Geometry check sheet. Reference: the model listing, model coordinates, mm. A direction names the side the tool comes from. Coordinates: 2 decimals unless noted, no trailing zeros. Order: outer loops, then holes, each group sorted by start corner. A loop starts at its lowest first (then second) coordinate and runs counter-clockwise, first axis right, second up. Notation, with made-up numbers: (6.25, 70.25) -> (40.25, 70.25) arc R22 ccw to (40.25, 108.25) -> close; hole circle Ø10 at (-28.75, 15). An arc over 180 degrees is marked (long way). Answer as CSV lines item,"result". Start each with the question number.
from build123d import *

# Parameters (mm, degrees)
BOSS_EXTRUDE1_DEPTH     = 40
CUT_EXTRUDE1_DEPTH      = 1.25
CUT_EXTRUDE1_DEPTH_BACK = 1.25


with BuildPart() as part:
    # Sketch1 → Boss-Extrude1 (new body)
    with BuildSketch(Plane.XY):
        with BuildLine():
            Line((-18.982831897, 2.385797253), (-16.305815663, 5.062813487))
            ThreePointArc((-16.305815663, 5.062813487), (-14.5, 0), (-16.305815663, -5.062813487))
            Line((-16.305815663, -5.062813487), (-18.982831897, -2.385797253))
            ThreePointArc((-18.982831897, -2.385797253), (-19.49479618, -3.00520382), (-20.114202747, -3.517168103))
            Line((-20.114202747, -3.517168103), (-16.01728135, -7.6140895))
            Line((-16.01728135, -7.6140895), (16.01728135, -7.6140895))
            Line((16.01728135, -7.6140895), (20.114202747, -3.517168103))
            ThreePointArc((20.114202747, -3.517168103), (19.49479618, -3.00520382), (18.982831897, -2.385797253))
            Line((18.982831897, -2.385797253), (16.305815663, -5.062813487))
            ThreePointArc((16.305815663, -5.062813487), (14.5, 0), (16.305815663, 5.062813487))
            Line((16.305815663, 5.062813487), (18.982831897, 2.385797253))
            ThreePointArc((18.982831897, 2.385797253), (19.49479618, 3.00520382), (20.114202747, 3.517168103))
            Line((20.114202747, 3.517168103), (17.437186513, 6.194184337))
            ThreePointArc((17.437186513, 6.194184337), (22.5, 8), (27.562813487, 6.194184337))
            Line((27.562813487, 6.194184337), (24.885797253, 3.517168103))
            ThreePointArc((24.885797253, 3.517168103), (25.50520382, 3.00520382), (26.017168103, 2.385797253))
            Line((26.017168103, 2.385797253), (28.694184337, 5.062813487))
            ThreePointArc((28.694184337, 5.062813487), (30.5, 0), (28.694184337, -5.062813487))
            Line((28.694184337, -5.062813487), (26.017168103, -2.385797253))
            ThreePointArc((26.017168103, -2.385797253), (25.50520382, -3.00520382), (24.885797253, -3.517168103))
            Line((24.885797253, -3.517168103), (28.98271865, -7.6140895))
            ThreePointArc((28.98271865, -7.6140895), (31.884585633, 3.453918427), (22.5, 10))
            Line((22.5, 10), (-22.5, 10))
            ThreePointArc((-22.5, 10), (-31.884585633, 3.453918427), (-28.98271865, -7.6140895))
            Line((-28.98271865, -7.6140895), (-24.885797253, -3.517168103))
            ThreePointArc((-24.885797253, -3.517168103), (-25.50520382, -3.00520382), (-26.017168103, -2.385797253))
            Line((-26.017168103, -2.385797253), (-28.694184337, -5.062813487))
            ThreePointArc((-28.694184337, -5.062813487), (-30.5, 0), (-28.694184337, 5.062813487))
            Line((-28.694184337, 5.062813487), (-26.017168103, 2.385797253))
            ThreePointArc((-26.017168103, 2.385797253), (-25.50520382, 3.00520382), (-24.885797253, 3.517168103))
            Line((-24.885797253, 3.517168103), (-27.562813487, 6.194184337))
            ThreePointArc((-27.562813487, 6.194184337), (-22.5, 8), (-17.437186513, 6.194184337))
            Line((-17.437186513, 6.194184337), (-20.114202747, 3.517168103))
            ThreePointArc((-20.114202747, 3.517168103), (-19.49479618, 3.00520382), (-18.982831897, 2.385797253))
        make_face()
    extrude(amount=BOSS_EXTRUDE1_DEPTH)

    # Sketch2 → Cut-Extrude1 (cut, two sides)
    with BuildSketch(Plane(origin=(0, 0, 0), x_dir=(0, 0, -1), z_dir=(1, 0, 0))) as cut_extrude1_sk:
        with BuildLine():
            Line((-40, 6), (-40, 8))
            ThreePointArc((-40, 8), (-38.585786438, 8.585786438), (-38, 10))
            Line((-38, 10), (-36, 10))
            ThreePointArc((-36, 10), (-37.171572875, 7.171572875), (-40, 6))
        make_face()
        with BuildLine():
            Line((-2, 10), (-4, 10))
            ThreePointArc((-4, 10), (-2.828427125, 7.171572875), (0, 6))
            Line((0, 6), (0, 8))
            ThreePointArc((0, 8), (-1.414213562, 8.585786438), (-2, 10))
        make_face()
    extrude(amount=CUT_EXTRUDE1_DEPTH, mode=Mode.SUBTRACT)
    extrude(cut_extrude1_sk.sketch, amount=-CUT_EXTRUDE1_DEPTH_BACK, mode=Mode.SUBTRACT)


solid = part.part
Q1. Sectioned sample at D-D, the plane y = 8.75. Record the cut outline in (x, z).
Q2. Sectioned sample at B-B, the plane y = 1. Record the cut outline in (x, z), then the cut area to 3 significant figures.
Q3. Sectioned sample at A-A, the plane x = 0. Record the cut outline in (y, z), then the cut area to 3 significant figures.
Q4. Go/stop test with flat-tipped pins: pin 1 Ø2 at (y, z) = (8.5, 37.5) entering from -X; pin 2 Ø4.5 at (y, z) = (7.5, 38.5) entering from +X; pin 3 Ø3 at (y, z) = (8.5, 1.5) entering from -X. Record where each tip stops, or that it passes through.
Q5. Thickness scan on L1, parallel to X at y = 0.5, z = 22.5; L2, parallel to X at y = 1.25, z = 22.5; L3, parallel to Y at x = 19, z = 12. Record the ranges inside material, lowest first.
Q6. Access from +Z, -Z, +X, -X, +Y, -Y to the whole of each face (thin tool, end or side, straight path). Record for faces 1 (the flat face through (-17.66, 3.71, 19.72)), 2 (the flat face through (0, 10, 20)), 3 (the flat face through (18.04, -5.59, 19.72)), 4 (the cylindrical face through (-0.018, 7.203, 37.141)).
Q7. Release check for a two-part mould opening along X. For faces 5 (the cylindrical face through (31.942, 3.293, 19.72)), 6 (the flat face through (-26.21, 4.84, 19.72)), 7 (the flat face through (26.91, -5.54, 19.72)), 8 (the flat face through (0, 1, 40)) record: released by +X, released by -X, zero draft, split by the parting line, or undercut.
Geometry results:
1,outline,"(-27.34, 0) -> (27.34, 0) -> (27.34, 40) -> (-27.34, 40) -> close; hole (-1.25, 1.56) -> (1.25, 1.56) -> (1.25, 3.8) -> (-1.25, 3.8) -> close; hole (-1.25, 36.2) -> (1.25, 36.2) -> (1.25, 38.44) -> (-1.25, 38.44) -> close"
2,outline,"(-32.45, 0) -> (-30.44, 0) -> (-30.44, 40) -> (-32.45, 40) -> close; (-14.56, 0) -> (14.56, 0) -> (14.56, 40) -> (-14.56, 40) -> close; (30.44, 0) -> (32.45, 0) -> (32.45, 40) -> (30.44, 40) -> close"
2,area,"1,330 mm^2"
3,outline,"(-7.61, 0) -> (6, 0) arc R4 cw to (10, 4) -> (10, 36) arc R4 cw to (6, 40) -> (-7.61, 40) -> close; (8, 0) -> (10, 0) -> (10, 2) arc R2 ccw to start; (8, 40) arc R2 ccw to (10, 38) -> (10, 40) -> close"
3,area,"686 mm^2"
4,pin 1,"stops at x = -29.11"
4,pin 2,"stops at x = 31.01"
4,pin 3,"stops at x = -29.64"
5,L1,"x = -32.49 to -30.48, -14.52 to 14.52, 30.48 to 32.49"
5,L2,"x = -32.42 to -30.4, -14.6 to 14.6, 30.4 to 32.42"
5,L3,"y = -4.63 to -2.41, 2.41 to 4.63, 7.19 to 10"
6,face 1,"+Z, -Z"
6,face 2,"+Z, -Z, +X, -X, +Y"
6,face 3,"+Z, -Z, -Y"
6,face 4,"none"
7,face 5,"released by +X"
7,face 6,"undercut"
7,face 7,"undercut"
7,face 8,"zero draft"
